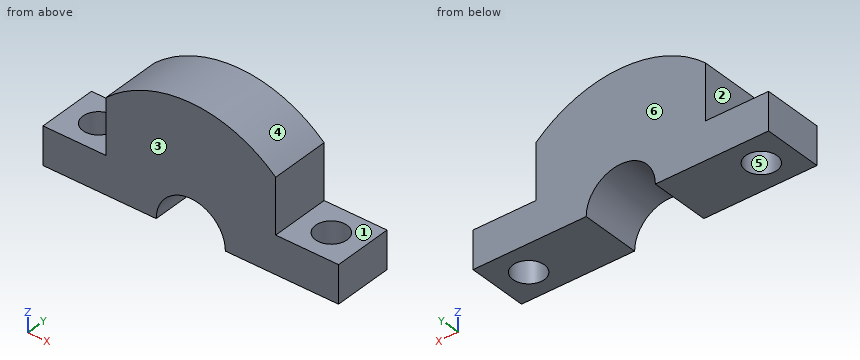
from build123d import *

# Parameters (mm, degrees)
F1_DEPTH = 4.75
F2_R     = 2.5
F3_DEPTH = 6.001


with BuildPart() as f1:
    # F0 (on Front) → F1 (new body, symmetric)
    with BuildSketch(Plane.XZ):
        with BuildLine():
            Line((-23.5, 6), (-23.5, 0))
            Line((-23.5, 0), (-5.5, 0))
            ThreePointArc((-5.5, 0), (0, 5.5), (5.5, 0))
            Line((5.5, 0), (23.5, 0))
            Line((23.5, 0), (23.5, 6))
            Line((23.5, 6), (13.5, 6))
            Line((13.5, 6), (13.5, 14.756355))
            ThreePointArc((13.5, 14.756355), (0, 20), (-13.5, 14.756355))
            Line((-13.5, 14.756355), (-13.5, 6))
            Line((-13.5, 6), (-23.5, 6))
        make_face()
    extrude(amount=F1_DEPTH, both=True)

    # F2 (on face) → F3 (cut, through all)
    with BuildSketch(Plane.XY.offset(6)):
        with Locations((-18.5, 0)):
            Circle(F2_R)
        with Locations((18.5, 0)):
            Circle(F2_R)
    extrude(amount=-F3_DEPTH, mode=Mode.SUBTRACT)


solid = f1.part
Source: CAD feature listing. Evaluate the final solid. Frame: model axes, mm. Face numbers are marked on the shaded views. A direction names the side the tool comes from. Coordinates: 2 decimals unless noted, no trailing zeros. Loops run counter-clockwise (first coordinate to the right, second up) from the corner with the lowest first, then second, coordinate; pieces in that order, holes last. Notation, with made-up numbers: (-17.75, 15.25) - (15.25, 15.25) arc R21 cw to (15.25, 19.25) - close; hole circle Ø1 at (12.5, 10). An arc over 180 degrees is marked (long way). Return JSON: item names as keys, results as strings.
Q1. Material intervals for line 1 along Y through (x, z) = (18.5, 2.45); line 2 along X through (y, z) = (-3.25, 4.25); line 3 along X through (y, z) = (1, 14.5), sorted ascending.
Results:
{"line 1": "-4.75 to -2.5, 2.5 to 4.75", "line 2": "-23.5 to -3.49, 3.49 to 23.5", "line 3": "-13.5 to 13.5"}
Q2. Section A-A, the plane x = -18.5. Return loops of the section in (y, z).
Results:
{"outline": "(-4.75, 0) - (-2.5, 0) - (-2.5, 6) - (-4.75, 6) - close; (2.5, 0) - (4.75, 0) - (4.75, 6) - (2.5, 6) - close"}
Q3. Contact query for flat-ended pins moving along their axis: P1, Ø4, axis at y = 1.5, z = 17.5, coming from the -X side; P2, Ø5, axis at y = 1, z = 9, coming from the +X side; P3, Ø5, axis at x = -18, y = -2, coming from the +Z side. Output: stop coordinate, or through.
Results:
{"P1": "x = -12.64", "P2": "x = 13.5", "P3": "z = 6"}
Q4. Section D-D, the plane y = -2. Return loops of the section in (x, z), plus the area to 3 significant figures.
Results:
{"outline": "(-23.5, 0) - (-20, 0) - (-20, 6) - (-23.5, 6) - close; (-17, 0) - (-5.5, 0) arc R5.5 cw to (5.5, 0) - (17, 0) - (17, 6) - (13.5, 6) - (13.5, 14.76) arc R20 ccw to (-13.5, 14.76) - (-13.5, 6) - (-17, 6) - close; (20, 0) - (23.5, 0) - (23.5, 6) - (20, 6) - close", "area": "532 mm2"}
Q5. Mould query, pull axis Y, two halves, no side actions, for the marked faces 4, 5 and 6. Classes: released by +Y, released by -Y, zero draft, split by the parting line, or undercut.
Results:
{"face 4": "zero draft", "face 5": "undercut", "face 6": "released by +Y"}
Q6. Section C-C, the plane z = 3.5. Return loops of the section in (x, y), plus the area to 3 significant figures.
Results:
{"outline": "(-23.5, -4.75) - (-4.24, -4.75) - (-4.24, 4.75) - (-23.5, 4.75) - close; (4.24, -4.75) - (23.5, -4.75) - (23.5, 4.75) - (4.24, 4.75) - close; hole circle Ø5 at (-18.5, 0); hole circle Ø5 at (18.5, 0)", "area": "327 mm2"}
Q7. Section B-B, the plane y = 0. Return loops of the section in (x, z), plus the area to 3 significant figures.
Results:
{"outline": "(-23.5, 0) - (-21, 0) - (-21, 6) - (-23.5, 6) - close; (-16, 0) - (-5.5, 0) arc R5.5 cw to (5.5, 0) - (16, 0) - (16, 6) - (13.5, 6) - (13.5, 14.76) arc R20 ccw to (-13.5, 14.76) - (-13.5, 6) - (-16, 6) - close; (21, 0) - (23.5, 0) - (23.5, 6) - (21, 6) - close", "area": "508 mm2"}
Q8. Access query for the marked faces 1, 2 and 3. Directions: +Z, -Z, +X, -X, +Y, -Y. A direction counts if a zero-diameter tool reaches every point of the face in a straight line with its end or side. Return the directions, or none.
Results:
{"face 1": "+Z, +X, +Y, -Y", "face 2": "+Z, -X, +Y, -Y", "face 3": "+Z, -Z, +X, -X, -Y"}
